For this review, use the dimensioned drawing (mm, ordinates from the lowest corner) and the shaded views. Round coordinates to 2 decimals unless told otherwise and drop trailing zeros. Write each loop counter-clockwise with the first axis right and the second up, starting at its lowest first coordinate (ties: lowest second). Pieces come first, ordered by that corner, then holes. Notation, with made-up numbers: M 75,61.5 L 104,61.5 A34 cw 104,93.5 Z; hole C -14,13.25 d10. An arc over 180 degrees is marked long. Use one line per item in the form item = value. Start each with the question number.
Item 1: Add section B-B (z = 28). State the section outline as (x, y) points (3 decimals).
Item 2: For P1, Ø5, axis at x = 8, z = 8.5, coming from the -Y side, flat-tipped, find the tip position at first contact; note if it passes through.
Item 3: Add section A-A (x = 28). State the section outline as (y, z) points.
Item 4: Add section D-D (y = 3.3). Count the separate pieces of the cut face and the enclosed holes in it, and give its area (3 significant figures).
Item 5: For line 1 (X direction, y = 2.95, z = 28) (3 decimals); line 2 (X direction, y = 2.95, z = 33.5); line 3 (Z direction, x = 86, y = 1.2), list the stretches that pass through material, from the lowest coordinate up. Write a range as [from, to].
Item 6: Add section C-C (x = 13). State the section outline as (y, z) points.
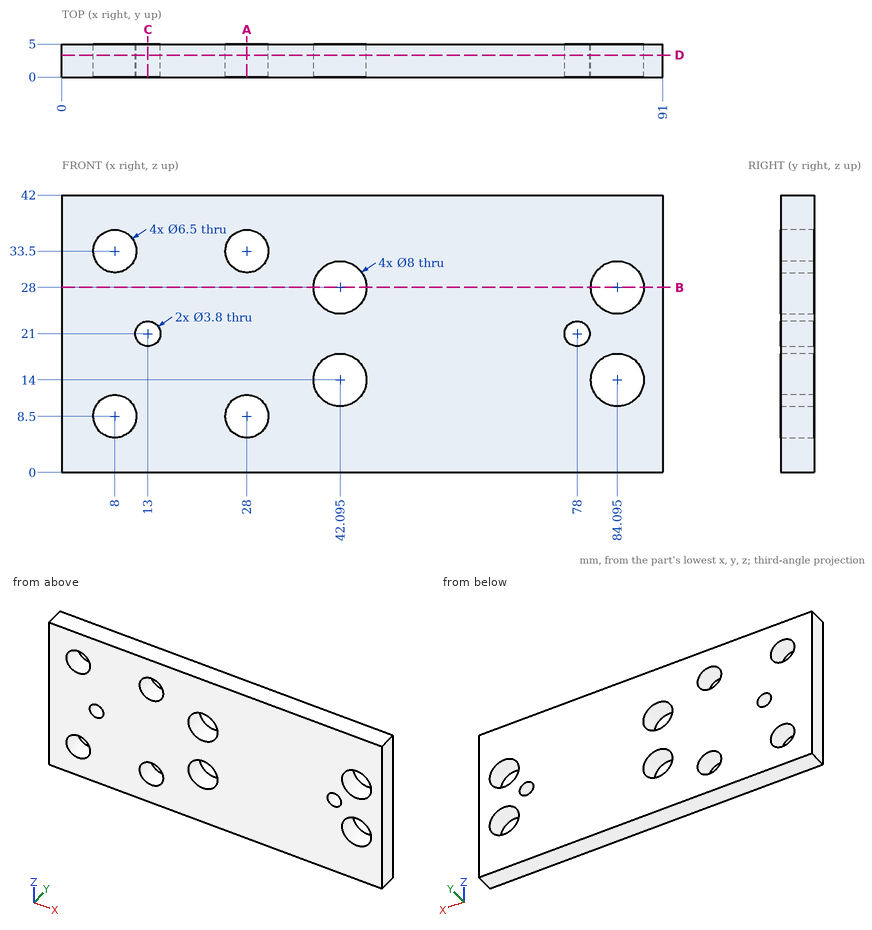
Calculated:
q1.outline = M 0,0 L 38.095,0 L 38.095,5 L 0,5 Z; M 46.095,0 L 80.095,0 L 80.095,5 L 46.095,5 Z; M 88.095,0 L 91,0 L 91,5 L 88.095,5 Z
q2.P1 = through
q3.outline = M 0,0 L 5,0 L 5,5.25 L 0,5.25 Z; M 0,11.75 L 5,11.75 L 5,30.25 L 0,30.25 Z; M 0,36.75 L 5,36.75 L 5,42 L 0,42 Z
q4.separate_pieces = 1
q4.enclosed_holes = 10
q4.area = 3,470 mm^2
q5.line_1 = [0, 38.095], [46.095, 80.095], [88.095, 91]
q5.line_2 = [0, 4.75], [11.25, 24.75], [31.25, 91]
q5.line_3 = [0, 10.48], [17.52, 24.48], [31.52, 42]
q6.outline = M 0,0 L 5,0 L 5,19.1 L 0,19.1 Z; M 0,22.9 L 5,22.9 L 5,42 L 0,42 Z
